from build123d import *

# Parameters (mm, degrees)
F0_R     = 19.05
F1_DEPTH = 6.35
F3_R     = 14.7955
F4_DEPTH = 6.35
F6_D     = 2.54


with BuildPart() as f1:
    # F0 (on Front) → F1 (new body)
    with BuildSketch(Plane.XZ):
        Circle(F0_R)
    extrude(amount=F1_DEPTH)

    # F3 (on offset) → F4 (join)
    with BuildSketch(Plane.XZ.offset(6.35)):
        Circle(F3_R)
    extrude(amount=F4_DEPTH)

    # F6 (through all)
    with Locations(Plane.XZ.offset(6.35)):
        with Locations((0, 17.124727), (15.2271, -7.064389), (-15.506332, -7.064389)):
            Hole(F6_D / 2)


solid = f1.part
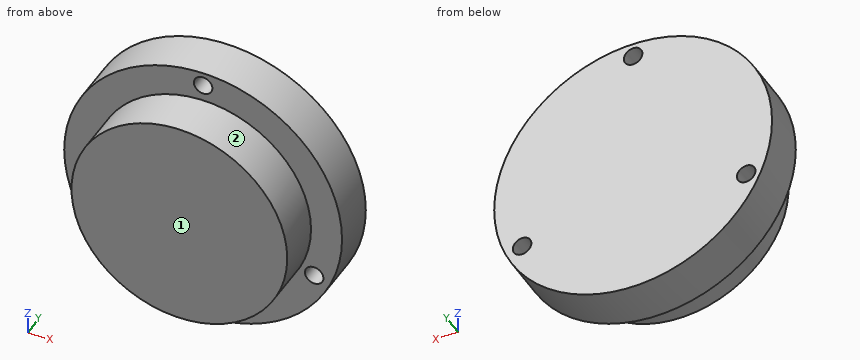
CAD build for the part. Positions are in the model's coordinates, mm. Face numbers are marked on the shaded views. A direction names the side the tool comes from. Coordinates: 2 decimals unless noted, no trailing zeros. Loops run counter-clockwise (first coordinate to the right, second up) from the corner with the lowest first, then second, coordinate; pieces in that order, holes last. Notation, with made-up numbers: (-13, 29.25) - (-7, 29.25) arc R21 cw to (-7, 68.25) - close; hole circle Ø7 at (38, 77). An arc over 180 degrees is marked (long way). Write item = value, one per line. Start each with the question number.
Q1. Cut at B-B, the plane z = 0. List the corners of the cut face in (x, y).
Q2. Cut at C-C, the plane y = -7.5. List the corners of the cut face in (x, z).
Q3. Which spindle directions (+Z, -Z, +X, -X, +Y, -Y) get a long thin tool onto all of the face, cutting with end or side? Do the marked faces 1 and 2. Say none if no direction does.
Q4. Drill centre lines: L1, parallel to X at y = -4.5, z = -6.5; L2, parallel to X at y = -0.25, z = -8; L3, parallel to Z at x = 0.5, y = -1.25. Where is each one in solid material? Low to high.
Q5. Flat gauge pins, fed straight in: pin 1 Ø3 at (x, z) = (-13, 14) entering from -Y; pin 2 Ø2 at (y, z) = (-10, -13.5) entering from -X; pin 3 Ø1 at (y, z) = (-11, -9) entering from +X. Where does each tip first touch, or does it go through?
Q6. Cut at A-A, the plane x = 0. List the corners of the cut face in (y, z).
Q7. Cut at D-D, the plane x = -8.5. List the corners of the cut face in (y, z).
Computed:
q1.outline = (-19.05, -6.35) - (-14.8, -6.35) - (-14.8, -12.7) - (14.8, -12.7) - (14.8, -6.35) - (19.05, -6.35) - (19.05, 0) - (-19.05, 0) - close
q2.outline = circle Ø29.59 at (0, 0)
q3.face_1 = +Z, -Z, +X, -X, -Y
q3.face_2 = -Y
q4.L1 = -17.91 to -16.64, -14.37 to 14.09, 16.36 to 17.91
q4.L2 = -17.29 to -16.37, -14.65 to 14.37, 16.09 to 17.29
q4.L3 = -19.04 to 15.96, 18.29 to 19.04
q5.pin_1 = -6.35
q5.pin_2 = -7.92
q5.pin_3 = 12.11
q6.outline = (-12.7, -14.8) - (-6.35, -14.8) - (-6.35, -19.05) - (0, -19.05) - (0, 15.85) - (-6.35, 15.85) - (-6.35, 14.8) - (-12.7, 14.8) - close; (-6.35, 18.39) - (0, 18.39) - (0, 19.05) - (-6.35, 19.05) - close
q7.outline = (-12.7, -12.11) - (-6.35, -12.11) - (-6.35, -17.05) - (0, -17.05) - (0, 17.05) - (-6.35, 17.05) - (-6.35, 12.11) - (-12.7, 12.11) - close
